Autodesk Fusion 360 part; units mm, degrees
sketch "Sketch1" plane through (0, 0, 0) normal (0, 0, 1) x (1, 0, 0)
  circle A0 centre (0, 0) radius 27.5
  circle A1 centre (0, 0) radius 35
  circle A2 centre (0, 0) radius 11.1
  circle A3 centre (0, 0) radius 8.6
  dimension "d1" = 55
  dimension "d2" = 70
  dimension "d3" = 22.2
  dimension "d4" = 17.2
extrude "Extrude1" add sketch "Sketch1" along normal blind 7.1 contours A2
extrude "Extrude2" add sketch "Sketch1" along normal blind 5 from surface at 7.1 contours A2 | A3
extrude "Extrude3" add sketch "Sketch1" along normal blind 5 contours A0 | A1
extrude "Extrude4" add sketch "Sketch1" along normal blind 12.1 contours A0
chamfer "Chamfer1" distance 5 angle 45 1 edges at (-25.639, -9.9444, 12.1)
extrude "Extrude5" cut sketch "Sketch1" along normal blind 7.1 contours A2
equation "d1 = SpoolHoleID"
equation "d2 = SpoolShelfOD"
equation "d3 = BearingOD"
equation "d4 = BearingOD - bearingHolderWallThickness"
equation "BearingOD = 22.20 mm"
equation "bearingHolderWallThickness = 5 mm"
equation "SpoolHoleID = 55 mm"
equation "SpoolShelfOD = 70 mm"
equation "SpoolShelfThickness = 5 mm"
equation "SpoolInsertHeight = 5 mm"
equation "SpoolInsertChamfer = 5 mm"
equation "BearingHeight = 7.10 mm"
equation "d13 = BearingHeight"
equation "d15 = BearingHeight"
equation "d16 = SpoolShelfThickness"
equation "d18 = SpoolShelfThickness"
equation "d20 = SpoolShelfThickness + BearingHeight"
equation "d22 = SpoolInsertChamfer"
equation "d23 = BearingHeight"
Build history of the part. All positions in model axes, mm. A direction names the side the tool comes from. Round coordinates to 2 decimals unless told otherwise and drop trailing zeros. Loops run counter-clockwise (first coordinate to the right, second up) from the corner with the lowest first, then second, coordinate; pieces in that order, holes last.
Item 1: Saw through at D-D (z = 10.5). List the corners of the cut face in (x, y).
Item 2: Drill centre lines: line 1 along Y through (x, z) = (0, 5.5); line 2 along Z through (x, y) = (-28, 10.5); line 3 along Z through (x, y) = (-4, -4.5). Where is each one in solid material? Low to high.
Item 3: Saw through at A-A (y = 0). List the corners of the cut face in (x, z), then the cut area to 3 significant figures.
Item 4: Which spindle directions (+Z, -Z, +X, -X, +Y, -Y) get a long thin tool onto all of the face, cutting with end or side? Do faces 1 (the face through (-21, -18, 5)), 2 (the face through (-8, 8, 0)). Say none if no direction does.
Item 5: Pin check, flat tips, straight feed: P1, Ø2, axis at x = 8, z = 3.5, coming from the -Y side; P2, Ø5, axis at y = 14, z = 2.5, coming from the -X side; P3, Ø18, axis at x = -2, y = -3, coming from the -Z side; P4, Ø2, axis at y = -6.5, z = 10.5, coming from the +X side. Stop position of each tip, or through.
Item 6: Saw through at C-C (z = 3). List the corners of the cut face in (x, y).
Item 7: Two-plate mould, pull along Y, no slides. Class faces 3 (the face through (5.97, -9.36, 3.5)), 4 (the face through (0, 0, 12.1)), 5 (the face through (-28, 21, 2)), 6 (the face through (0, 0, 7.1)): released by +Y, released by -Y, zero draft, split by the parting line, or undercut.
Worked answers:
1. outline: circle Ø48.2 at (0, 0)
2. line 1: y = -27.5 to -11.1, 11.1 to 27.5
2. line 2: z = 0 to 5
2. line 3: z = 7.1 to 12.1
3. outline: (-35, 0) - (-11.1, 0) - (-11.1, 7.1) - (11.1, 7.1) - (11.1, 0) - (35, 0) - (35, 5) - (27.5, 5) - (27.5, 7.1) - (22.5, 12.1) - (-22.5, 12.1) - (-27.5, 7.1) - (-27.5, 5) - (-35, 5) - close
3. area: 558 mm2
4. face 1: +Z
4. face 2: -Z, +X, -X, +Y, -Y
5. P1: stops at y = -34.29
5. P2: stops at x = -33.06
5. P3: stops at z = 0
5. P4: stops at x = 24.28
6. outline: circle Ø70 at (0, 0); hole circle Ø22.2 at (0, 0)
7. face 3: undercut
7. face 4: zero draft
7. face 5: split by the parting line
7. face 6: undercut
